CAD build for the part. Positions are in the model's coordinates, mm. A direction names the side the tool comes from. Round coordinates to 2 decimals unless told otherwise and drop trailing zeros. Order: outer loops, then holes, each group sorted by start corner. A loop starts at its lowest first (then second) coordinate and runs counter-clockwise, first axis right, second up. Notation, with made-up numbers: M 17,26 L 45,26 A28 cw 45,48 Z; hole C 41,9.5 d8. An arc over 180 degrees is marked long. Answer as a JSON object with one key per item and string values. Group by question number.
```python
from build123d import *

# Parameters (mm, degrees)
SKETCH1_W            = 1.75
SKETCH1_H            = 4.1
BOSS_EXTRUDE1_DEPTH  = 1.6
BOSS_EXTRUDE2_DEPTH  = 2
SKETCH3_W            = 1
SKETCH3_H            = 0.6
BOSS_EXTRUDE3_DEPTH  = 1.8
SKETCH4_W            = 1
SKETCH4_H            = 0.6
BOSS_EXTRUDE4_DEPTH  = 2.25
BOSS_EXTRUDE5_DEPTH  = 1
SKETCH6_W            = 4.1
SKETCH6_H            = 4
BOSS_EXTRUDE6_DEPTH  = 0.65
SKETCH7_W            = 2
SKETCH7_H            = 0.6
BOSS_EXTRUDE7_DEPTH  = 2
SKETCH8_W            = 4.1
SKETCH8_H            = 6
BOSS_EXTRUDE8_DEPTH  = 0.65
SKETCH9_W            = 5.9
SKETCH9_H            = 6
BOSS_EXTRUDE9_DEPTH  = 0.4
SKETCH10_W           = 0.8
SKETCH10_H           = 1.9
CUT_EXTRUDE1_DEPTH   = 1.65
SKETCH11_W           = 0.8
SKETCH11_H           = 1.9
CUT_EXTRUDE2_DEPTH   = 6.9
SKETCH12_W           = 0.5
SKETCH12_H           = 0.5
BOSS_EXTRUDE10_DEPTH = 3.3
SKETCH13_W           = 0.5
SKETCH13_H           = 0.5
BOSS_EXTRUDE11_DEPTH = 3.3
SKETCH14_W           = 0.5
SKETCH14_H           = 0.5
BOSS_EXTRUDE12_DEPTH = 1.5
SKETCH15_W           = 0.5
SKETCH15_H           = 0.5
BOSS_EXTRUDE13_DEPTH = 1.5


with BuildPart() as part:
    # Sketch1 → Boss-Extrude1 (new body)
    with BuildSketch(Plane(origin=(4.6, 0, 0), x_dir=(0, -1, 0), z_dir=(-1, 0, 0))):
        with Locations((-0.875, 2.45)):
            Rectangle(SKETCH1_W, SKETCH1_H)
    extrude(amount=-BOSS_EXTRUDE1_DEPTH)

    # Sketch2 → Boss-Extrude2 (add)
    with BuildSketch(Plane(origin=(6.2, 0, 0), x_dir=(0, 0, -1), z_dir=(1, 0, 0))):
        Polygon((-3.9, 1.75), (-0.4, 1.75), (-0.4, 0), (-4.5, 0), (-4.5, 2.2), (-3.9, 2.2), align=None)
    extrude(amount=BOSS_EXTRUDE2_DEPTH)

    # Sketch3 → Boss-Extrude3 (add)
    with BuildSketch(Plane(origin=(0, 2.2, 0), x_dir=(-1, 0, 0), z_dir=(0, 1, 0))):
        with Locations((-6.7, 4.2)):
            Rectangle(SKETCH3_W, SKETCH3_H)
    extrude(amount=BOSS_EXTRUDE3_DEPTH)

    # Sketch4 → Boss-Extrude4 (add)
    with BuildSketch(Plane(origin=(0, 1.75, 0), x_dir=(-1, 0, 0), z_dir=(0, 1, 0))):
        with Locations((-5.1, 4.2)):
            Rectangle(SKETCH4_W, SKETCH4_H)
    extrude(amount=BOSS_EXTRUDE4_DEPTH)

    # Sketch5 → Boss-Extrude5 (add)
    with BuildSketch(Plane.ZY.offset(-4.6)):
        Polygon((0.4, 0), (0.4, 1.75), (3.9, 1.75), (3.9, 2.2), (4.5, 2.2), (4.5, 0), align=None)
    extrude(amount=BOSS_EXTRUDE5_DEPTH)

    # Sketch6 → Boss-Extrude6 (add)
    with BuildSketch(Plane.ZY.offset(-3.6)):
        with Locations((2.45, 2)):
            Rectangle(SKETCH6_W, SKETCH6_H)
    extrude(amount=BOSS_EXTRUDE6_DEPTH)

    # Sketch7 → Boss-Extrude7 (add)
    with BuildSketch(Plane(origin=(0, 4, 0), x_dir=(-1, 0, 0), z_dir=(0, 1, 0))):
        with Locations((-7.2, 4.2)):
            Rectangle(SKETCH7_W, SKETCH7_H)
        Polygon((-3.6, 0.4), (-3.6, 3.9), (-5.6, 3.9), (-5.6, 4.5), (-2.95, 4.5), (-2.95, 0.4), align=None)
    extrude(amount=BOSS_EXTRUDE7_DEPTH)

    # Sketch8 → Boss-Extrude8 (add)
    with BuildSketch(Plane(origin=(8.2, 0, 0), x_dir=(0, 0, -1), z_dir=(1, 0, 0))):
        with Locations((-2.45, 3)):
            Rectangle(SKETCH8_W, SKETCH8_H)
    extrude(amount=BOSS_EXTRUDE8_DEPTH)

    # Sketch9 → Boss-Extrude9 (add)
    with BuildSketch(Plane(origin=(0, 0, 0.4), x_dir=(-1, 0, 0), z_dir=(0, 0, -1))):
        with Locations((-5.9, 3)):
            Rectangle(SKETCH9_W, SKETCH9_H)
    extrude(amount=BOSS_EXTRUDE9_DEPTH)

    # Sketch10 → Cut-Extrude1 (cut, through all)
    with BuildSketch(Plane(origin=(3.6, 0, 0), x_dir=(0, 0, -1), z_dir=(1, 0, 0))):
        with Locations((-2.65, 5.05)):
            Rectangle(SKETCH10_W, SKETCH10_H)
    extrude(amount=-CUT_EXTRUDE1_DEPTH, mode=Mode.SUBTRACT)

    # Sketch11 → Cut-Extrude2 (cut, through all)
    with BuildSketch(Plane(origin=(8.85, 0, 0), x_dir=(0, 0, -1), z_dir=(1, 0, 0))):
        with Locations((-2.65, 5.05)):
            Rectangle(SKETCH11_W, SKETCH11_H)
    extrude(amount=-CUT_EXTRUDE2_DEPTH, mode=Mode.SUBTRACT)

    # Sketch12 → Boss-Extrude10 (add)
    with BuildSketch(Plane(origin=(0, 1.75, 0), x_dir=(-1, 0, 0), z_dir=(0, 1, 0))):
        with Locations((-4.9, 2.8)):
            Rectangle(SKETCH12_W, SKETCH12_H)
    extrude(amount=BOSS_EXTRUDE10_DEPTH)

    # Sketch13 → Boss-Extrude11 (add)
    with BuildSketch(Plane(origin=(0, 1.75, 0), x_dir=(-1, 0, 0), z_dir=(0, 1, 0))):
        with Locations((-6.9, 2.8)):
            Rectangle(SKETCH13_W, SKETCH13_H)
    extrude(amount=BOSS_EXTRUDE11_DEPTH)

    # Sketch14 → Boss-Extrude12 (add)
    with BuildSketch(Plane.XZ):
        with Locations((4.9, 2.8)):
            Rectangle(SKETCH14_W, SKETCH14_H)
    extrude(amount=BOSS_EXTRUDE12_DEPTH)

    # Sketch15 → Boss-Extrude13 (add)
    with BuildSketch(Plane.XZ):
        with Locations((6.9, 2.8)):
            Rectangle(SKETCH15_W, SKETCH15_H)
    extrude(amount=BOSS_EXTRUDE13_DEPTH)


solid = part.part
```
Item 1: 3-axis set-ups, long thin cutter, end or side, ignore diameter. For faces 1 (the face through (4, 6, 4.1)), 2 (the face through (5, 4, 3.9)): which of +Z, -Z, +X, -X, +Y, -Y reach the whole face in a straight line?
Item 2: Drill centre lines: line 1 (X direction, y = 5.5, z = 3.45); line 2 (Z direction, x = 4.6, y = 4.5); line 3 (Y direction, x = 5.65, z = 3.7). Where is each one in solid material? Low to high. Write a range as [from, to].
Item 3: Cut at D-D, the plane z = 4. Give the cut face in (x, y).
Item 4: Cut at C-C, the plane y = -0.5. Give the cut face in (x, z).
Item 5: Two-plate mould, pull along X, no slides. Class faces 3 (the face through (7, 3, 4.5)), 4 (the face through (8.2, 4, 2)), 5 (the face through (8.85, 3, 2)): +X half, -X half, draft (parallel to the pull), parting line (faces both ways), or undercut.
Item 6: Cut at A-A, the plane y = 4.75. Give the cut face in (x, z), and give its area (3 significant figures).
Item 7: Flat gauge pins, fed straight in: pin 1 Ø1.5 at (x, y) = (5.5, 4) entering from -Z; pin 2 Ø0.6 at (x, y) = (7, -0.5) entering from -Z; pin 3 Ø0.6 at (y, z) = (-1, 3) entering from +X; pin 4 Ø1 at (x, z) = (7.5, 1) entering from +Y. Where does each tip first touch, or does it go through?
Item 8: Cut at B-B, the plane x = 3.85. Give the cut face in (y, z).
Response values:
{
 "1": {"face 1": "+Z, -Z, +X, -X, +Y", "face 2": "+Y"},
 "2": {"line 1": "[2.95, 3.6], [8.2, 8.85]", "line 2": "[0, 0.4], [3.9, 4.5]", "line 3": "[0, 1.75]"},
 "3": {"outline": "M 2.95,0 L 8.85,0 L 8.85,6 L 6.2,6 L 6.2,1.75 L 5.6,1.75 L 5.6,6 L 2.95,6 Z; hole M 3.6,2.2 L 4.6,2.2 L 4.6,4 L 3.6,4 Z; hole M 7.2,2.2 L 8.2,2.2 L 8.2,4 L 7.2,4 Z"},
 "4": {"outline": "M 4.65,2.55 L 5.15,2.55 L 5.15,3.05 L 4.65,3.05 Z; M 6.65,2.55 L 7.15,2.55 L 7.15,3.05 L 6.65,3.05 Z"},
 "5": {"face 3": "draft", "face 4": "undercut", "face 5": "+X half"},
 "6": {"outline": "M 2.95,0 L 8.85,0 L 8.85,2.25 L 8.2,2.25 L 8.2,0.4 L 3.6,0.4 L 3.6,2.25 L 2.95,2.25 Z; M 2.95,3.05 L 3.6,3.05 L 3.6,3.9 L 5.6,3.9 L 5.6,4.5 L 2.95,4.5 Z; M 4.65,2.55 L 5.15,2.55 L 5.15,3.05 L 4.65,3.05 Z; M 6.2,3.9 L 8.2,3.9 L 8.2,3.05 L 8.85,3.05 L 8.85,4.5 L 6.2,4.5 Z; M 6.65,2.55 L 7.15,2.55 L 7.15,3.05 L 6.65,3.05 Z", "area": "9.55 mm^2"},
 "7": {"pin 1": "z = 0", "pin 2": "z = 2.55", "pin 3": "x = 7.15", "pin 4": "y = 1.75"},
 "8": {"outline": "M 0,0 L 6,0 L 6,0.4 L 1.75,0.4 L 1.75,3.9 L 2.2,3.9 L 2.2,4.5 L 0,4.5 Z; M 4,3.9 L 6,3.9 L 6,4.5 L 4,4.5 Z"}
}
